Source: CAD feature listing. Evaluate the final solid. Frame: model axes, mm. Face numbers are marked on the shaded views. A direction names the side the tool comes from. Give positions to 0.01 mm unless a question says otherwise; leave off trailing zeros. Loops run counter-clockwise (first coordinate to the right, second up) from the corner with the lowest first, then second, coordinate; pieces in that order, holes last. Notation, with made-up numbers: M 14.5,47.25 L 61.5,47.25 A17 ccw 61.5,69.25 Z; hole C 37,71.5 d2. An arc over 180 degrees is marked long. Put each result on its own line as item: value.
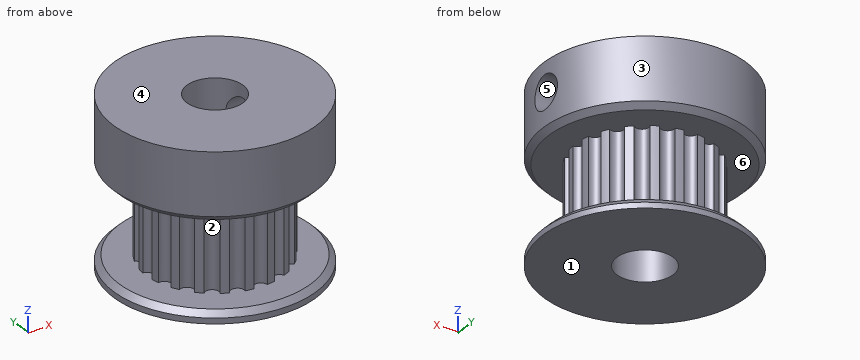
from build123d import *

# Parameters (mm, degrees)
CYLINDER014_R           = 1.5
CYLINDER014_DEPTH       = 9
CYLINDER014_PITCH_ANGLE = 90
CYLINDER013_R           = 2.5
CYLINDER013_DEPTH       = 14.6
CYLINDER011_R           = 9
CYLINDER011_DEPTH       = 1
CHAMFER007_SIZE         = 0.5
CYLINDER012_R           = 9
CYLINDER012_DEPTH       = 6
CHAMFER008_SIZE         = 0.5
CYLINDER009_R           = 0.6
CYLINDER009_DEPTH       = 7.6
ARRAY_COUNT             = 20
CYLINDER010_R           = 6.1
CYLINDER010_DEPTH       = 7.6


with BuildPart() as cilindro007:
    # Cylinder014 → Cylinder014 (new body)
    with BuildSketch(Plane.XY):
        Circle(CYLINDER014_R)
    extrude(amount=CYLINDER014_DEPTH)


with BuildPart() as cilindro007_1:
    # Cylinder014 pitch: moved
    add(cilindro007.part.rotate(Axis((0, 0, 0), (0, 1, 0)), CYLINDER014_PITCH_ANGLE))


with BuildPart() as cilindro007_2:
    # Cylinder014 placement: moved
    add(cilindro007_1.part.moved(Location((1, 0, 12))))


with BuildPart() as cilindro006:
    # Cylinder013 → Cylinder013 (new body)
    with BuildSketch(Plane.XY):
        Circle(CYLINDER013_R)
    extrude(amount=CYLINDER013_DEPTH)


with BuildPart() as chamfer007:
    # Cylinder011 → Cylinder011 (new body)
    with BuildSketch(Plane.XY):
        Circle(CYLINDER011_R)
    extrude(amount=CYLINDER011_DEPTH)

    # Chamfer007
    chamfer007_edges = [chamfer007.edges().sort_by_distance(p)[0] for p in [
        (-9, 0, 1),
    ]]
    chamfer(chamfer007_edges, length=CHAMFER007_SIZE)


with BuildPart() as chamfer008:
    # Cylinder012 → Cylinder012 (new body)
    with BuildSketch(Plane.XY.offset(8.6)):
        Circle(CYLINDER012_R)
    extrude(amount=CYLINDER012_DEPTH)

    # Chamfer008
    chamfer008_edges = [chamfer008.edges().sort_by_distance(p)[0] for p in [
        (-9, 0, 8.6),
    ]]
    chamfer(chamfer008_edges, length=CHAMFER008_SIZE)


with BuildPart() as array:
    # Cylinder009 → Cylinder009 (new body)
    with BuildSketch(Plane(origin=(6.1, 0, 0), x_dir=(1, 0, 0), z_dir=(0, 0, 1))):
        Circle(CYLINDER009_R)
    extrude(amount=CYLINDER009_DEPTH)

    # Array: Array ×20 about axis
    array_axis = Axis((0, 0, 0), (0, 0, 1))


with BuildPart() as array_1:
    add(array.part)
    for i in range(1, ARRAY_COUNT):
        add(array.part.rotate(array_axis, i * 360 / ARRAY_COUNT))


with BuildPart() as cut017:
    # Cylinder010 → Cylinder010 (new body)
    with BuildSketch(Plane.XY):
        Circle(CYLINDER010_R)
    extrude(amount=CYLINDER010_DEPTH)

    # Cut015: cut Array
    add(array_1.part, mode=Mode.SUBTRACT)


with BuildPart() as cut017_1:
    # Cut015 placement: moved
    add(cut017.part.moved(Location((0, 0, 1))))

    # Fusion006: union Chamfer007, Chamfer008
    add(chamfer007.part)
    add(chamfer008.part)

    # Cut016: cut Cilindro006
    add(cilindro006.part, mode=Mode.SUBTRACT)

    # Cut017: cut Cilindro007
    add(cilindro007_2.part, mode=Mode.SUBTRACT)


solid = cut017_1.part
1. Material intervals for line 1 (Z direction, x = 7.5, y = 0); line 2 (Y direction, x = 0, z = 10.25); line 3 (Z direction, x = 4.25, y = -5.25), sorted ascending. Write a range as from..to.
Found:
line 1: 0..1, 8.6..10.5, 13.5..14.6
line 2: -9..-2.5, 2.5..9
line 3: 0..1, 8.6..14.6
2. Contact query for flat-ended pins moving along their axis: P1, Ø5, axis at x = 6.5, y = -6, coming from the -Z side; P2, Ø2, axis at x = -6, z = 8.5, coming from the +Y side. Output: stop coordinate, or through.
Found:
P1: z = 0
P2: y = 7.35
3. Access query for the marked faces 4, 5 and 6. Directions: +Z, -Z, +X, -X, +Y, -Y. A direction counts if a zero-diameter tool reaches every point of the face in a straight line with its end or side. Return the directions, or none.
Found:
face 4: +Z, +X, -X, +Y, -Y
face 5: +X
face 6: none
4. Section query C-C (z = 12). Output: boundary loops of the cut face in (x, y).
Found:
outline: M 2,-1.5 A2.5 cw long 2,1.5 L 8.87,1.5 A9 ccw long 8.87,-1.5 Z
5. Draft query along Y for the marked faces 1, 2 and 3. Return one class per face: pulls with the +Y half, pulls with the -Y half, needs draft (parallel to the pull), parting line crosses it, or undercut.
Found:
face 1: needs draft
face 2: undercut
face 3: parting line crosses it
6. Section query A-A (y = 0). Output: boundary loops of the cut face in (x, z), plus the area to 3 significant figures.
Found:
outline: M -9,0 L -2.5,0 L -2.5,14.6 L -9,14.6 L -9,9.1 L -8.5,8.6 L -5.5,8.6 L -5.5,1 L -8.5,1 L -9,0.5 Z; M 2.5,0 L 9,0 L 9,0.5 L 8.5,1 L 5.5,1 L 5.5,8.6 L 8.5,8.6 L 9,9.1 L 9,10.5 L 2.5,10.5 Z; M 2.5,13.5 L 9,13.5 L 9,14.6 L 2.5,14.6 Z
area: 117 mm^2
7. Section query B-B (x = 7.5). State how many separate pieces and enclosed holes the cut face has, plus the area to 3 significant figures.
Found:
separate pieces: 2
enclosed holes: 1
area: 61.6 mm^2
